Here's how the part is built. I have some questions about the finished solid (model axes, mm). A direction names the side the tool comes from. Coordinates: 2 decimals unless noted, no trailing zeros. Write each loop counter-clockwise with the first axis right and the second up, starting at its lowest first coordinate (ties: lowest second). Pieces come first, ordered by that corner, then holes.
Item 1: For faces 5 (the face through (66, -53, 6)), 6 (the face through (65.29, -50.22, 3.97)), 7 (the face through (68.19, 46.42, 3.97)), 8 (the face through (-30.346, 24, 17)), 9 (the face through (-69, 47, 6)), which set-ups out of +Z, -Z, +X, -X, +Y, -Y let a thin tool reach every point of the face, with its end or its side?
Item 2: I'm going to push flat-ended pins straight in: pin 1 Ø6.5 at (y, z) = (20.5, 17) entering from -X; pin 2 Ø6 at (y, z) = (1.5, 14) entering from -X; pin 3 Ø11 at (y, z) = (21.5, 7) entering from +X; pin 4 Ø3.5 at (x, y) = (67, 48) entering from +Z. Where does each tip first touch, or does it pass through?
Item 3: If we section it at A-A (x = -1.5): Please give me the cut outline in (y, z), then the cut area to 3 significant figures.
Item 4: We'd pull the mould along Y, two halves only. Please class faces 1 (the face through (-75.4, -0.8, 1.5)), 2 (the face through (0, 40.604, 17)), 3 (the face through (-68, 48, 2)), 4 (the face through (0, 8.604, 17)): +Y half, -Y half, draft (parallel to the pull), parting line (faces both ways), or undercut.
Item 5: If I drill on line 1 (Y direction, x = 67.5, z = 12.9); line 2 (X direction, y = -29.5, z = 5.5); line 3 (Y direction, x = -67.5, z = 4.85), over which ranges is the centre line in solid material (lowest first)?
Item 6: If we section it at B-B (y = 10.5): Please give me the cut outline in (x, z).
Item 7: If we section it at C-C (x = 51): Please give me the cut outline in (y, z), then the cut area to 3 significant figures.
from build123d import *

# Parameters (mm, degrees)
SKETCH_1_W          = 153.8
SKETCH_1_H          = 120
SKETCH_1_W_2        = 113.5
SKETCH_1_H_2        = 85.5
EXTRUDE_1_DEPTH     = 6
CHAMFER_1_SIZE      = 3
SHELL_1_T           = -2
SKETCH_3_W          = 121.15685425
SKETCH_3_H          = 93.15685425
CUT_EXTRUDE_1_DEPTH = 4
SKETCH_4_R          = 3
SKETCH_4_R_2        = 1.5
EXTRUDE_3_DEPTH     = 4
SKETCH_2_W          = 123
SKETCH_2_H          = 102
EXTRUDE_2_DEPTH     = 10
SKETCH_5_W          = 145
SKETCH_5_H          = 111
EXTRUDE_4_DEPTH     = 1.6
CUT_EXTRUDE_START   = -1.6
SKETCH_6_R          = 1.5
CUT_EXTRUDE_2_DEPTH = 1.6
SKETCH_7_W          = 61
SKETCH_7_H          = 32
EXTRUDE_5_DEPTH     = 6


with BuildPart() as part:
    # 草图1 → 凸台-拉伸1 (new body)
    with BuildSketch(Plane.XY):
        Rectangle(SKETCH_1_W, SKETCH_1_H)
        with Locations((0, -2.25)):
            Rectangle(SKETCH_1_W_2, SKETCH_1_H_2, mode=Mode.SUBTRACT)
    extrude(amount=EXTRUDE_1_DEPTH)

    # 倒角1
    chamfer_1_edges = [part.edges().sort_by_distance(p)[0] for p in [
        (56.75, -2.25, 0),
        (0, 40.5, 0),
        (-56.75, -2.25, 0),
        (0, -45, 0),
        (0, 60, 0),
        (76.9, 0, 0),
        (0, -60, 0),
        (-76.9, 0, 0),
    ]]
    chamfer(chamfer_1_edges, length=CHAMFER_1_SIZE)

    # 抽壳1
    shell_1_openings = [part.faces().sort_by_distance(p)[0] for p in [
        (0, 58.049245274, 6),
    ]]
    offset(amount=SHELL_1_T, openings=shell_1_openings, kind=Kind.INTERSECTION)

    # 草图3 → 切除-拉伸1 (cut)
    with BuildSketch(Plane.XY.offset(6)):
        with Locations((0, -2.25)):
            Rectangle(SKETCH_3_W, SKETCH_3_H)
    extrude(amount=-CUT_EXTRUDE_1_DEPTH, mode=Mode.SUBTRACT)

    # 草图4 → 凸台-拉伸3 (add)
    # profile 1 of 4: a face of its own
    with BuildSketch(Plane.XY.offset(2)):
        with Locations((-67.5, 47.75)):
            Circle(SKETCH_4_R)
        with Locations((-67.5, 47.75)):
            Circle(SKETCH_4_R_2, mode=Mode.SUBTRACT)
    # profile 2 of 4: a face of its own
    with BuildSketch(Plane.XY.offset(2)):
        with Locations(Location((67.5, 47.75, 0), (0, 0, 180))):
            Circle(SKETCH_4_R)
        with Locations((67.5, 47.75)):
            Circle(SKETCH_4_R_2, mode=Mode.SUBTRACT)
    # profile 3 of 4: a face of its own
    with BuildSketch(Plane.XY.offset(2)):
        with Locations((67.5, -52.25)):
            Circle(SKETCH_4_R)
        with Locations((67.5, -52.25)):
            Circle(SKETCH_4_R_2, mode=Mode.SUBTRACT)
    # profile 4 of 4: a face of its own
    with BuildSketch(Plane.XY.offset(2)):
        with Locations(Location((-67.5, -52.25, 0), (0, 0, 180))):
            Circle(SKETCH_4_R)
        with Locations((-67.5, -52.25)):
            Circle(SKETCH_4_R_2, mode=Mode.SUBTRACT)
    extrude(amount=EXTRUDE_3_DEPTH)

    # 草图2 → 凸台-拉伸2 (add)
    with BuildSketch(Plane.XY.offset(2)):
        with Locations((0, -2.25)):
            Rectangle(SKETCH_2_W, SKETCH_2_H)
    extrude(amount=EXTRUDE_2_DEPTH)

    # 草图5 → 凸台-拉伸4 (add)
    with BuildSketch(Plane.XY.offset(12)):
        with Locations((0, -2.25)):
            Rectangle(SKETCH_5_W, SKETCH_5_H)
    extrude(amount=EXTRUDE_4_DEPTH)

    # 草图6 → 切除-拉伸2 (cut)
    with BuildSketch(Plane.XY.offset(13.6).offset(CUT_EXTRUDE_START)):
        with Locations((-67.5, 47.75)):
            Circle(SKETCH_6_R)
        with Locations((67.5, 47.75)):
            Circle(SKETCH_6_R)
        with Locations((67.5, -52.25)):
            Circle(SKETCH_6_R)
        with Locations((-67.5, -52.25)):
            Circle(SKETCH_6_R)
    extrude(amount=CUT_EXTRUDE_2_DEPTH, mode=Mode.SUBTRACT)

    # 草图7 → 凸台-拉伸5 (add)
    with BuildSketch(Plane.XY.offset(13.6)):
        with Locations((0.153519833, 24.604445294)):
            Rectangle(SKETCH_7_W, SKETCH_7_H)
    extrude(amount=EXTRUDE_5_DEPTH)


solid = part.part
Answer list:
1. face 5: +X, +Y, -Y
1. face 6: none
1. face 7: +Z
1. face 8: +Z, -X, +Y, -Y
1. face 9: -X, +Y, -Y
2. pin 1: stops at x = -30.35
2. pin 2: stops at x = -72.5
2. pin 3: stops at x = 76.9
2. pin 4: stops at z = 13.6
3. outline: (-60, 3) - (-57, 0) - (-48, 0) - (-46, 2) - (41.5, 2) - (43.5, 0) - (57, 0) - (60, 3) - (60, 6) - (58, 6) - (58, 3.83) - (56.17, 2) - (48.75, 2) - (48.75, 12) - (53.25, 12) - (53.25, 13.6) - (40.6, 13.6) - (40.6, 19.6) - (8.6, 19.6) - (8.6, 13.6) - (-57.75, 13.6) - (-57.75, 12) - (-53.25, 12) - (-53.25, 2) - (-56.17, 2) - (-58, 3.83) - (-58, 6) - (-60, 6) - close
3. area: 1,460 mm2
4. face 1: draft
4. face 2: +Y half
4. face 3: undercut
4. face 4: -Y half
5. line 1: y = -57.75 to -53.75, -50.75 to 46.25, 49.25 to 53.25
5. line 2: x = -76.9 to -74.9, -61.5 to 61.5, 74.9 to 76.9
5. line 3: y = -60 to -58, -55.25 to -53.75, -50.75 to -49.25, 44.75 to 46.25, 49.25 to 50.75, 58 to 60
6. outline: (-76.9, 3) - (-73.9, 0) - (-59.75, 0) - (-57.75, 2) - (57.75, 2) - (59.75, 0) - (73.9, 0) - (76.9, 3) - (76.9, 6) - (74.9, 6) - (74.9, 3.83) - (73.07, 2) - (61.5, 2) - (61.5, 12) - (72.5, 12) - (72.5, 13.6) - (30.65, 13.6) - (30.65, 19.6) - (-30.35, 19.6) - (-30.35, 13.6) - (-72.5, 13.6) - (-72.5, 12) - (-61.5, 12) - (-61.5, 2) - (-73.07, 2) - (-74.9, 3.83) - (-74.9, 6) - (-76.9, 6) - close
7. outline: (-60, 3) - (-57, 0) - (-48, 0) - (-46, 2) - (41.5, 2) - (43.5, 0) - (57, 0) - (60, 3) - (60, 6) - (58, 6) - (58, 3.83) - (56.17, 2) - (48.75, 2) - (48.75, 12) - (53.25, 12) - (53.25, 13.6) - (-57.75, 13.6) - (-57.75, 12) - (-53.25, 12) - (-53.25, 2) - (-56.17, 2) - (-58, 3.83) - (-58, 6) - (-60, 6) - close
7. area: 1,270 mm2
